Here's how the part is built. I have some questions about the finished solid (model axes, mm). A direction names the side the tool comes from. Round coordinates to 2 decimals unless told otherwise and drop trailing zeros. Write each loop counter-clockwise with the first axis right and the second up, starting at its lowest first coordinate (ties: lowest second). Pieces come first, ordered by that corner, then holes. Notation, with made-up numbers: (-8.75, 31.25) -> (48.25, 31.25) arc R28 cw to (48.25, 52.25) -> close; hole circle Ø5 at (20.25, -17.75). An arc over 180 degrees is marked (long way). Answer in a Markdown table with one row per item.
Autodesk Inventor part; units mm, degrees
ref_plane "YZ Plane" through (0, 0, 0) normal (1, 0, 0) x (0, 1, 0)
ref_plane "XZ Plane" through (0, 0, 0) normal (0, 1, 0) x (-1, 0, 0)
ref_plane "XY Plane" through (0, 0, 0) normal (0, 0, 1) x (1, 0, 0)
sketch "Sketch1" plane through (0, 0, 0) normal (0, 0, 1) x (1, 0, 0)
  arc A0 (-56.515, 0) -> (56.515, 0) centre (0, 0) ccw
  line L0 (114.3, -88.9) -> (-114.3, -88.9)
  line L1 (-114.3, 88.9) -> (114.3, 88.9) construction
  line L2 (-56.515, 0) -> (-114.3, 0)
  line L3 (-114.3, -76.2) -> (-81.5672, -76.2)
  line L4 (81.5672, -76.2) -> (114.3, -76.2)
  line L5 (114.3, 0) -> (114.3, -12.7)
  line L6 (114.3, -76.2) -> (114.3, -88.9)
  line L7 (-114.3, -88.9) -> (-114.3, -76.2)
  line L8 (-114.3, -12.7) -> (-114.3, 0)
  line L9 (-114.3, 0) -> (-56.515, 0)
  line L10 (56.515, 0) -> (114.3, 0)
  line L11 (-114.3, -12.7) -> (-81.5672, -12.7)
  line L12 (81.5672, -12.7) -> (114.3, -12.7)
  line L13 (-81.5672, -12.7) -> (-81.5672, -76.2)
  line L14 (81.5672, -12.7) -> (81.5672, -76.2)
  dimension "d0" = 113.03
  dimension "d7" = 57.785
extrude "Extrusion1" add sketch "Sketch1" along normal blind 25.4
sketch "Sketch2" plane through (81.5672, -12.7, 0) normal (0, -1, 0) x (1, 0, 0)
  line L0 (32.7328, 0) -> (0, 25.4) construction
  line L1 (-195.8672, 0) -> (-195.8672, 25.4)
  line L2 (-195.8672, 25.4) -> (-163.1345, 0) construction
  point P0 (-81.5672, 0)
  point P1 (-179.5008, 12.7)
  point P2 (16.3664, 12.7)
hole "Hole1" at (-97.9336, -12.7, 12.7) at (97.9336, -12.7, 12.7) direction (0, -1, 0) diameter 6.604 end through all
sketch "Sketch3" plane through (-114.3, -88.9, 0) normal (0, -1, 0) x (1, 0, 0)
  circle A0 centre (212.2336, 12.7) radius 3.302
  circle A1 centre (16.3664, 12.7) radius 3.302
  point P0 (114.3, 0)
hole "Hole2" at (97.9336, -88.9, 12.7) at (-97.9336, -88.9, 12.7) direction (0, 1, 0) diameter 6.7564 end through all
sketch "Sketch4" plane through (-114.3, -12.7, 0) normal (0, -1, 0) x (1, 0, 0)
  circle A0 centre (16.3664, 12.7) radius 3.3782
  circle A1 centre (16.3664, 12.7) radius 4.318
  circle A2 centre (212.2336, 12.7) radius 3.3782
  circle A3 centre (212.2336, 12.7) radius 4.318
  point P0 (114.3, 0)
  dimension "d26" = 8.636
  dimension "d27" = 8.636
extrude "Extrusion2" cut sketch "Sketch4" against normal blind 8.382
chamfer "Chamfer1" distance 3.175 angle 45 6 edges at (-56.515, 0, 12.7) (56.515, 0, 12.7) (-114.3, -6.35, 25.4) (-114.3, -6.35, 0) (114.3, -6.35, 25.4) (114.3, -6.35, 0)
chamfer "Chamfer2" distance 3.175 angle 45 18 edges at (0, -56.515, 25.4) (0, -56.515, 0) (-81.5672, -44.45, 25.4) (-96.3461, -12.7, 25.4) (-81.5672, -44.45, 0) (-96.3461, -12.7, 0) (-114.3, -12.7, 12.7) (-97.9336, -76.2, 25.4) (-97.9336, -76.2, 0) (-114.3, -76.2, 12.7) (81.5672, -44.45, 25.4) (81.5672, -44.45, 0) (96.3461, -12.7, 25.4) (114.3, -12.7, 12.7) (96.3461, -12.7, 0) (97.9336, -76.2, 25.4) (114.3, -76.2, 12.7) (97.9336, -76.2, 0)
properties part number "2121_Copper Tube Clamp Bottom_V1" material "ABS Plastic"
1) I want a section at A-A, the plane y = -65. List the corners of the cut face in (x, z) for me (3 decimals).
Response:
| item | result |
|---|---|
| outline | (-81.567, 3.175) -> (-78.392, 0) -> (78.392, 0) -> (81.567, 3.175) -> (81.567, 22.225) -> (78.392, 25.4) -> (-78.392, 25.4) -> (-81.567, 22.225) -> close |
2) I want a section at C-C, the plane x = 0. List the corners of the cut face in (y, z) for me (3 decimals).
Response:
| item | result |
|---|---|
| outline | (-88.9, 0) -> (-59.69, 0) -> (-56.515, 3.175) -> (-56.515, 22.225) -> (-59.69, 25.4) -> (-88.9, 25.4) -> close |
3) Which directions (+Z, -Z, +X, -X, +Y, -Y) give clear straight access to the entire face, cutting with the end or side of a thin tool? Please do faces 4 (the face through (93, -12.7, 13)), 5 (the face through (-102.247, -8.568, 12.89)), 6 (the face through (-87, 0, 13)), 7 (the face through (-93, -76.2, 13)).
Response:
| item | result |
|---|---|
| face 4 | +Z, -Z, +X |
| face 5 | none |
| face 6 | +Z, -Z, +X, -X, +Y |
| face 7 | +Z, -Z, -X |
4) For pin 1 (8 mm diameter, centred on y = -20.5, z = 19, fed in from +X); pin 2 (10 mm diameter, centred on x = -21.5, z = 14, fed in from +Y); pin 3 (6 mm diameter, centred on y = -13, z = 8.5, fed in from +X) (3 decimals), each with a flat end and sliding along its axis, tell me the tip position at first contact or that it passes through.
Response:
| item | result |
|---|---|
| pin 1 | stops at x = 81.57 |
| pin 2 | stops at y = -49.92 |
| pin 3 | stops at x = 113.825 |
5) I want a section at B-B, the plane z = 12.7. Count the separate pieces of the cut face and the enclosed holes in it, and give its area (3 significant figures).
Response:
| item | result |
|---|---|
| separate pieces | 5 |
| enclosed holes | 0 |
| area | 10,700 mm^2 |
6) I need wall thicknesses on line 1 (X direction, y = -85, z = 12); line 2 (Y direction, x = -89, z = 7.25); line 3 (X direction, y = -71, z = 8.5). Which ranges of each line are inside material? Lowest first, please. Write a range as [from, to].
Response:
| item | result |
|---|---|
| line 1 | x = [-114.3, -101.24], [-94.63, 94.63], [101.24, 114.3] |
| line 2 | y = [-88.9, -76.2], [-12.7, 0] |
| line 3 | x = [-81.57, 81.57] |
7) We'd pull the mould along X, two halves only. Please class faces 1 (the face through (-94.937, -2.129, 11.141)), 2 (the face through (81.567, -44, 13)), 3 (the face through (-93, -12.7, 13)): +X half, -X half, draft (parallel to the pull), parting line (faces both ways), or undercut.
Response:
| item | result |
|---|---|
| face 1 | undercut |
| face 2 | +X half |
| face 3 | draft |
